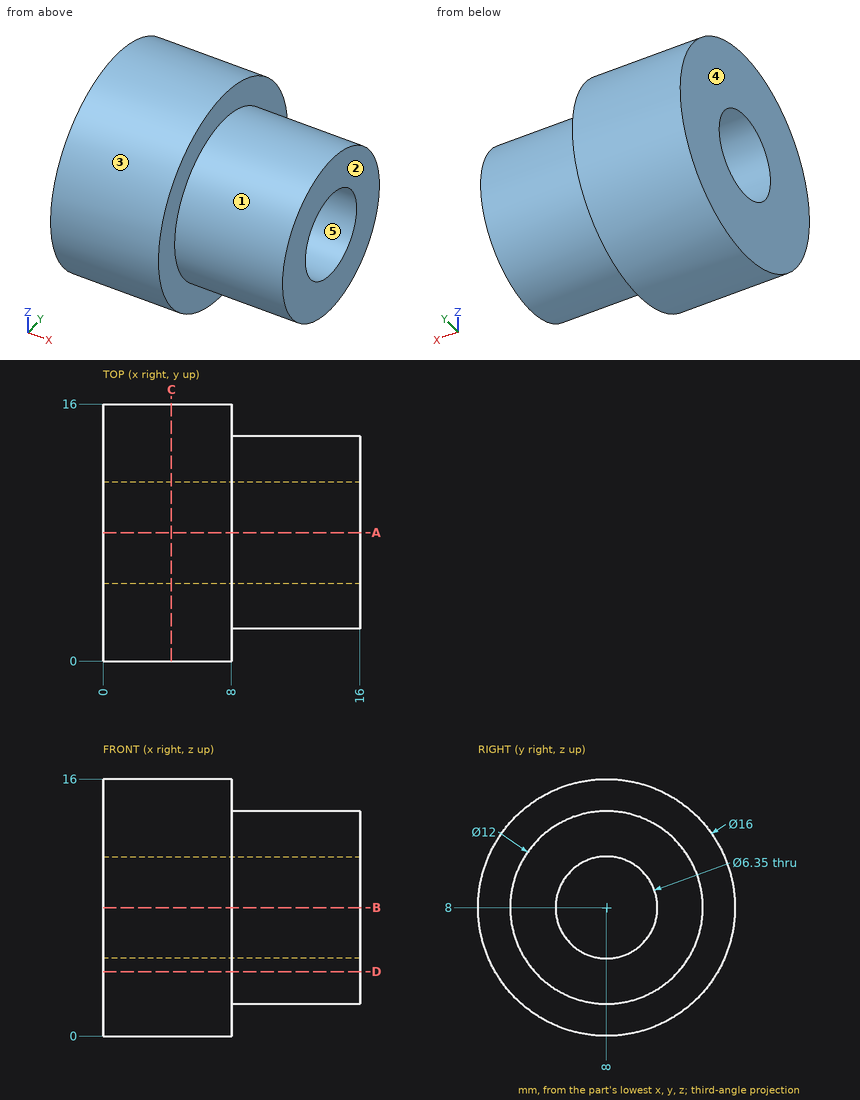
Geometry check sheet. Reference: drawing and pictorial views, mm from the part's lowest x, y, z. A direction names the side the tool comes from. Coordinates: 2 decimals unless noted, no trailing zeros. Write each loop counter-clockwise with the first axis right and the second up, starting at its lowest first coordinate (ties: lowest second). Pieces come first, ordered by that corner, then holes. Notation, with made-up numbers: (-32, -2) - (-13, -2) arc R21 ccw to (-13, 27) - close; hole circle Ø1 at (31.25, 30.25). An arc over 180 degrees is marked (long way). Write item = value, one per line.
Q1. Cross-section at D-D (z = 4). Enter the section's corners in (x, y), plus the area to 3 significant figures.
Answer:
outline = (0, 1.07) - (8, 1.07) - (8, 3.53) - (16, 3.53) - (16, 12.47) - (8, 12.47) - (8, 14.93) - (0, 14.93) - close
area = 182 mm²
Q2. Go/stop test with flat-tipped pins: pin 1 Ø8 at (x, y) = (9, 13.5) entering from -Z; pin 2 Ø1 at (x, z) = (6, 10) entering from +Y; pin 3 Ø1.5 at (x, z) = (5, 11) entering from +Y; pin 4 Ø6 at (y, z) = (8.5, 8) entering from -X. Record where each tip stops, or that it passes through.
Answer:
pin_1 = 0.17
pin_2 = 15.86
pin_3 = 15.68
pin_4 = 0
Q3. Access from +Z, -Z, +X, -X, +Y, -Y to the whole of each face (thin tool, end or side, straight path). Record for the marked faces 1 and 2.
Answer:
face_1 = +X
face_2 = +Z, -Z, +X, +Y, -Y
Q4. Cross-section at C-C (x = 4.25). Enter the section's corners in (y, z) (3 decimals).
Answer:
outline = circle Ø16 at (8, 8); hole circle Ø6.35 at (8, 8)
Q5. Material ranges on L1, parallel to X at y = 13, z = 13; L2, parallel to Y at x = 9, z = 8 (3 decimals); L3, parallel to Y at x = 6.25, z = 8 (3 decimals), recorded low to high. Write a range as from..to.
Answer:
L1 = 0..8
L2 = 2..4.825, 11.175..14
L3 = 0..4.825, 11.175..16
Q6. Mould release check, pull along Y, two halves, no side actions. Record for the marked faces 3, 4 and 5: released by +Y, released by -Y, zero draft, split by the parting line, or undercut.
Answer:
face_3 = split by the parting line
face_4 = zero draft
face_5 = undercut
Q7. Cross-section at A-A (y = 8). Enter the section's corners in (x, z) (3 decimals).
Answer:
outline = (0, 0) - (8, 0) - (8, 2) - (16, 2) - (16, 4.825) - (0, 4.825) - close; (0, 11.175) - (16, 11.175) - (16, 14) - (8, 14) - (8, 16) - (0, 16) - close
